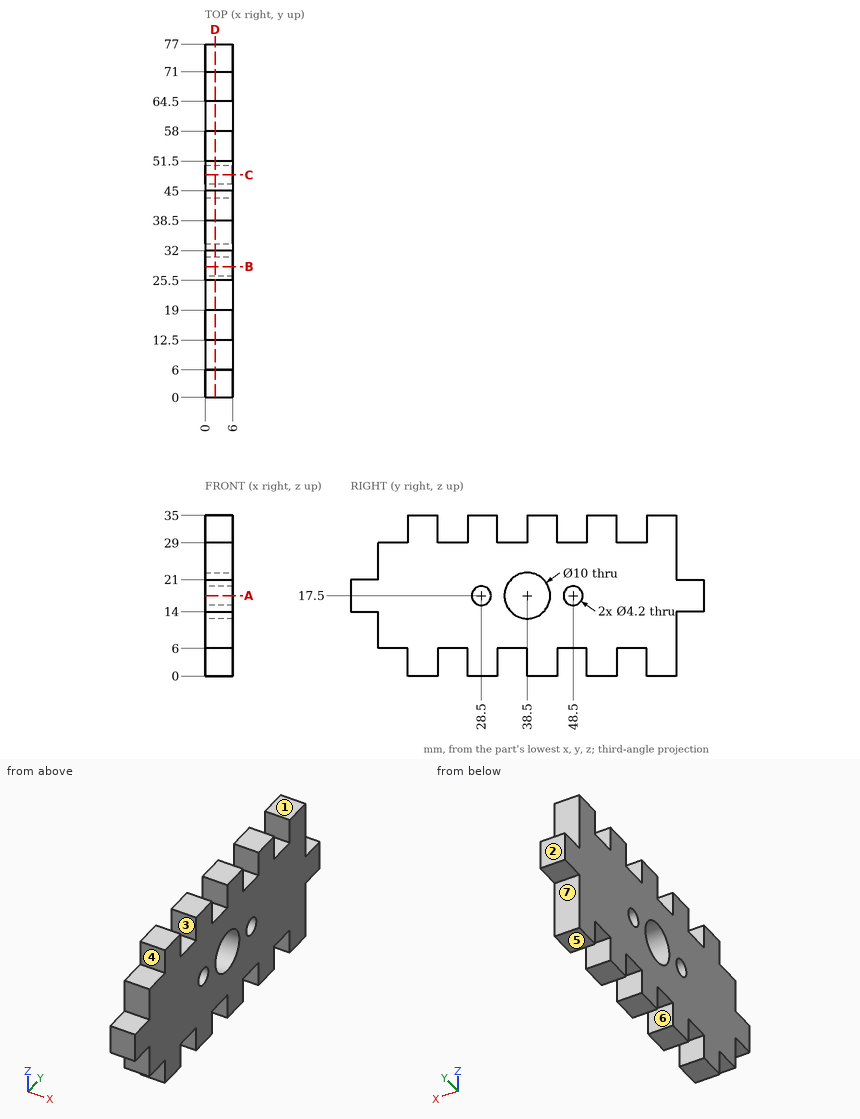
Source: three-view drawing plus pictorial views. Frame: mm from the lowest corner of the part. A direction names the side the tool comes from. Coordinates: 2 decimals unless noted, no trailing zeros. Order: outer loops, then holes, each group sorted by start corner. A loop starts at its lowest first (then second) coordinate and runs counter-clockwise, first axis right, second up.
1) Set-up query: the marked faces 4, 5, 6 and 7. Return all of +Z, -Z, +X, -X, +Y, -Y with unobstructed straight access to the full face (end or side cutting, diameter ignored); none if empty.
Result sheet:
face 4: +Z, +X, -X, -Y
face 5: -Z, +X, -X, +Y, -Y
face 6: -Z, +X, -X
face 7: -Z, +X, -X, +Y
2) Section B-B (y = 28.5). Return loops of the section in (x, z), then the cut area to 3 significant figures.
Result sheet:
outline: (0, 0) - (6, 0) - (6, 15.4) - (0, 15.4) - close; (0, 19.6) - (6, 19.6) - (6, 35) - (0, 35) - close
area: 185 mm2
3) Section D-D (x = 2.2). Give the number of separate pieces and of enclosed holes in the cut face, then the cut area to 3 significant figures.
Result sheet:
separate pieces: 1
enclosed holes: 3
area: 1,860 mm2
4) Ray query, probe 1 along Y at (x, z) = (3.3, 5.5); probe 2 along Z at (x, y) = (2.95, 28.5); probe 3 along Z at (x, y) = (3.1, 48.5). Return the intervals inside material, ascending.
Result sheet:
probe 1: y = 12.5 to 19, 25.5 to 32, 38.5 to 45, 51.5 to 58, 64.5 to 71
probe 2: z = 0 to 15.4, 19.6 to 35
probe 3: z = 6 to 15.4, 19.6 to 29
5) Draft query along Y for the marked faces 1, 2 and 3. Return one class per face: released by +Y, released by -Y, zero draft, split by the parting line, or undercut.
Result sheet:
face 1: zero draft
face 2: released by +Y
face 3: undercut
6) Section A-A (z = 17.5). Return loops of the section in (x, y), then the cut area to 3 significant figures.
Result sheet:
outline: (0, 0) - (6, 0) - (6, 26.4) - (0, 26.4) - close; (0, 30.6) - (6, 30.6) - (6, 33.5) - (0, 33.5) - close; (0, 43.5) - (6, 43.5) - (6, 46.4) - (0, 46.4) - close; (0, 50.6) - (6, 50.6) - (6, 77) - (0, 77) - close
area: 352 mm2
7) Section C-C (y = 48.5). Return loops of the section in (x, z).
Result sheet:
outline: (0, 6) - (6, 6) - (6, 15.4) - (0, 15.4) - close; (0, 19.6) - (6, 19.6) - (6, 29) - (0, 29) - close
8) First-contact query: P1, Ø1.8, axis at x = 1.5, z = 4.5, coming from the -Y side; P2, Ø3, axis at x = 1.5, z = 12, coming from the -Y side; P3, Ø3, axis at x = 3.5, z = 32.5, coming from the +Y side. Flat tips, straight axial feed; report the tip coordinate or a pass-through.
Result sheet:
P1: stops at y = 12.5
P2: stops at y = 6
P3: stops at y = 71
